from build123d import *

# Parameters (mm, degrees)
F1_DEPTH = 12.7
F4_W     = 25.4
F4_H     = 25.4
F3_W     = 25.4
F3_H     = 50.8
F6_W     = 25.4
F6_H     = 25.4
F7_DEPTH = 25.4


with BuildPart() as f1:
    # F0 (on Right) → F1 (new body, symmetric)
    with BuildSketch(Plane.YZ):
        Polygon((-50.8, 0), (0, 0), (0, 25.4), (-25.4, 25.4), align=None)
    extrude(amount=F1_DEPTH, both=True)

    # F4 (on face) → F5 section 0
    with BuildSketch(Plane(origin=(-12.7, 0, 0), x_dir=(0, -1, 0), z_dir=(-1, 0, 0))):
        with Locations((12.7, 12.7)):
            Rectangle(F4_W, F4_H)
    # F3 (on offset) → F5 section 1
    with BuildSketch(Plane.YZ.offset(-63.5)):
        with Locations((-12.7, 25.4)):
            Rectangle(F3_W, F3_H)
    loft()

    # F6 (on face) → F7 (join)
    with BuildSketch(Plane.XZ.offset(25.4)):
        with Locations((-50.8, 12.7)):
            Rectangle(F6_W, F6_H)
    extrude(amount=F7_DEPTH)


solid = f1.part
Model file for the job. Use its own axes, mm. A direction names the side the tool comes from. Round coordinates to 2 decimals unless told otherwise and drop trailing zeros. Order: outer loops, then holes, each group sorted by start corner. A loop starts at its lowest first (then second) coordinate and runs counter-clockwise, first axis right, second up. Notation, with made-up numbers: M 20,18.5 L 52,18.5 A22 cw 52,38.5 Z; hole C 77.5,-36 d1. An arc over 180 degrees is marked long. Write each question's results on one line, items separated by ' | '. Start each with the question number.
(1) Saw through at B-B, the plane y = -16.5. Give the cut face in (x, z), then the cut area to 3 significant figures.
(2) Saw through at A-A, the plane y = -42. Give the cut face in (x, z).
(3) Drop flat-ended pins along their axis: pin 1 (1 mm diameter, centred on x = -4, y = -10, fed in from +Z); pin 2 (12 mm diameter, centred on x = -11, z = 32.5, fed in from +Y). Give the stop position or say it passes through.
(4) Saw through at C-C, the plane y = -31.5. Give the cut face in (x, z).
(5) Saw through at D-D, the plane x = 0. Give the cut face in (y, z).
(6) Probe probe 1 along X at (y, z) = (-29, 18.5); probe 2 along Z at (x, y) = (-3, -20); probe 3 along Y at (x, z) = (-52, 34.5). List the from-to ranges inside material, lowest first. Write a range as from..to.
(7) Which spindle directions (+Z, -Z, +X, -X, +Y, -Y) get a long thin tool onto all of the face, cutting with end or side? Do faces 5 (the face through (0, -13, 25.4)), 6 (the face through (0.2, -37.9, 12.9)), 7 (the face through (-31, 0, 16)). Say none if no direction does.
(8) Two-plate mould, pull along X, no slides. Class faces 1 (the face through (-63.5, -19, 19)), 2 (the face through (-12.7, -33, 7)), 3 (the face through (-38.1, -38, 13)), 4 (the face through (-51, -38, 25.4)): pulls with the +X half, pulls with the -X half, needs draft (parallel to the pull), parting line crosses it, or undercut.
Established:
1) outline: M -63.5,0 L 12.7,0 L 12.7,25.4 L -12.7,25.4 L -63.5,50.8 Z | area: 2,580 mm^2
2) outline: M -63.5,0 L -38.1,0 L -38.1,25.4 L -63.5,25.4 Z; M -12.7,0 L 12.7,0 L 12.7,8.8 L -12.7,8.8 Z
3) pin 1: stops at z = 25.4 | pin 2: passes through
4) outline: M -63.5,0 L -38.1,0 L -38.1,25.4 L -63.5,25.4 Z; M -12.7,0 L 12.7,0 L 12.7,19.3 L -12.7,19.3 Z
5) outline: M -50.8,0 L 0,0 L 0,25.4 L -25.4,25.4 Z
6) probe 1: x = -63.5..-38.1, -12.7..12.7 | probe 2: z = 0..25.4 | probe 3: y = -25.4..0
7) face 5: +Z, +X, +Y, -Y | face 6: +Z, +X, -Y | face 7: +Z, -Z, +X, -X, +Y
8) face 1: pulls with the -X half | face 2: undercut | face 3: undercut | face 4: needs draft
